```python
from build123d import *

# Parameters (mm, degrees)
BOSS_EXTRUDE1_DEPTH     = 6
SKETCH2_R               = 2.1
CUT_EXTRUDE1_DEPTH      = 41.755367745
CUT_EXTRUDE2_DEPTH      = 10
CUT_EXTRUDE2_DEPTH_BACK = 10
SKETCH3_W               = 25
SKETCH3_H               = 2
FILLET5_R               = 1


with BuildPart() as part:
    # Sketch1 → Boss-Extrude1 (new body)
    with BuildSketch(Plane.XY):
        with BuildLine():
            ThreePointArc((35, -5), (30, 0), (35, 5))
            Line((35, 5), (-35, 5))
            ThreePointArc((-35, 5), (-31.464466094, 3.535533906), (-30, 0))
            ThreePointArc((-30, 0), (-31.464466094, -3.535533906), (-35, -5))
            Line((-35, -5), (35, -5))
        make_face()
        with BuildLine():
            ThreePointArc((-30, 0), (-31.464466094, 3.535533906), (-35, 5))
            ThreePointArc((-35, 5), (-40, 0), (-35, -5))
            ThreePointArc((-35, -5), (-31.464466094, -3.535533906), (-30, 0))
        make_face()
        with BuildLine():
            ThreePointArc((40, 0), (38.535533906, 3.535533906), (35, 5))
            ThreePointArc((35, 5), (30, 0), (35, -5))
            ThreePointArc((35, -5), (38.535533906, -3.535533906), (40, 0))
        make_face()
    extrude(amount=BOSS_EXTRUDE1_DEPTH)

    # Sketch2 → Cut-Extrude1 (cut, through all)
    with BuildSketch(Plane.XY.offset(6)):
        with Locations((-35, 0)):
            Circle(SKETCH2_R)
        with Locations(Location((35, 0, 0), (0, 0, 180))):
            Circle(SKETCH2_R)
    extrude(amount=-CUT_EXTRUDE1_DEPTH, mode=Mode.SUBTRACT)

    # Sketch3 → Cut-Extrude2 (cut, two sides: drawn at the far end of the back side and taken through both)
    with BuildSketch(Plane(origin=(0, 0, 0), x_dir=(1, 0, 0), z_dir=(0, 1, 0)).offset(-CUT_EXTRUDE2_DEPTH_BACK)):
        with Locations((-40, -3)):
            Rectangle(SKETCH3_W, SKETCH3_H)
        with Locations((40, -3)):
            Rectangle(SKETCH3_W, SKETCH3_H)
    extrude(amount=CUT_EXTRUDE2_DEPTH + CUT_EXTRUDE2_DEPTH_BACK, mode=Mode.SUBTRACT)

    # SurfaceCut1
    split(bisect_by=Plane.XY.offset(3), keep=Keep.BOTTOM)

    # Mirror12: part across plane


with BuildPart() as part_1:
    add(part.part)
    add(part.part.mirror(Plane.XY.offset(3)))

    # Fillet5
    fillet5_edges = [part_1.edges().sort_by_distance(p)[0] for p in [
        (-27.5, 0, 2),
        (27.5, 0, 2),
        (27.5, 0, 4),
        (-27.5, 0, 4),
    ]]
    fillet(fillet5_edges, radius=FILLET5_R - 0.0001)  # a hair under: the kernel refuses the full size


solid = part_1.part
```
Geometry: final body of the model. Coordinates: model frame, mm. A direction names the side the tool comes from. Round coordinates to 2 decimals unless told otherwise and drop trailing zeros. Order: outer loops, then holes, each group sorted by start corner. A loop starts at its lowest first (then second) coordinate and runs counter-clockwise, first axis right, second up. Notation, with made-up numbers: (-13.5, 18.5) -> (26.5, 18.5) arc R26 ccw to (26.5, 33.5) -> close; hole circle Ø11 at (-1.5, 17). An arc over 180 degrees is marked (long way). Use one line per item in the form item = value.
(1) Access query for faces 1 (the face through (0, -5, 3)), 2 (the face through (-33.05, -1.18, 2)). Directions: +Z, -Z, +X, -X, +Y, -Y. A direction counts if a zero-diameter tool reaches every point of the face in a straight line with its end or side. Return the directions, or none.
Results list:
face_1 = +Z, -Z, +X, -X, -Y
face_2 = -X, +Y, -Y
(2) First-contact query: pin 1 Ø3 at (y, z) = (3.5, 1.5) entering from +X. Flat tip, straight axial feed; report the tip coordinate or a pass-through.
Results list:
pin_1 = 39.58
(3) Draft query along Z for faces 3 (the face through (32.9, 1, 2)), 4 (the face through (-1, 0, 6)), 5 (the face through (32.9, 1, 4)), 6 (the face through (-40, 0, 5)). Return one class per face: pulls with the +Z half, pulls with the -Z half, needs draft (parallel to the pull), parting line crosses it, or undercut.
Results list:
face_3 = undercut
face_4 = pulls with the +Z half
face_5 = undercut
face_6 = needs draft
(4) Section A-A on x = 32. Return loops of the section in (y, z), and give its area (3 significant figures).
Results list:
outline = (-5, 0) -> (5, 0) -> (5, 2) -> (-5, 2) -> close; (-5, 4) -> (5, 4) -> (5, 6) -> (-5, 6) -> close
area = 40.0 mm^2
(5) Ray query, probe 1 along Y at (x, z) = (-35, 1.45); probe 2 along Z at (x, y) = (35.5, -2.5); probe 3 along X at (y, z) = (1.75, 4.95). Return the intervals inside material, ascending. Write a range as [from, to].
Results list:
probe_1 = [-5, -2.1], [2.1, 5]
probe_2 = [0, 2], [4, 6]
probe_3 = [-39.68, -36.16], [-33.84, 33.84], [36.16, 39.68]
(6) Section B-B on z = 4.85. Return loops of the section in (x, y).
Results list:
outline = (-35, -5) -> (35, -5) arc R5 ccw to (35, 5) -> (-35, 5) arc R5 ccw to start; hole circle Ø4.2 at (-35, 0); hole circle Ø4.2 at (35, 0)
